from build123d import *

# Parameters (mm, degrees)
F0_R     = 25.4
F2_R     = 15.875
F4_R     = 15.875
F5_DEPTH = 50.8
F6_R     = 5.08
F7_DEPTH = 25.4
F8_DEPTH = 50.8
F9_R     = 5.08


with BuildPart() as f3:
    # F0 (on Top) → F3 section 0
    with BuildSketch(Plane.XY):
        Circle(F0_R)
    # F2 (on offset) → F3 section 1
    with BuildSketch(Plane.XY.offset(50.8)):
        Circle(F2_R)
    loft()

    # F4 (on face) → F5 (join)
    with BuildSketch(Plane.XY.offset(50.8)):
        Circle(F4_R)
    extrude(amount=F5_DEPTH)

    # F6 (on Front) → F7 (join)
    with BuildSketch(Plane.XZ):
        with Locations((0, 79.9094587564)):
            Circle(F6_R)
    extrude(amount=F7_DEPTH)

    # F8 (add): a face of the model
    f8_faces = [f3.faces().sort_by_distance(p)[0] for p in [
        (0, -25.4, 79.9094587564),
    ]]
    extrude(f8_faces, amount=-F8_DEPTH)

    # F9
    f9_edges = [f3.edges().sort_by_distance(p)[0] for p in [
        (-15.875, 0, 101.6),
    ]]
    fillet(f9_edges, radius=F9_R)

    # F10 (on Front) → F11 (revolve)
    with BuildSketch(Plane.XZ):
        Polygon((-15.8836290712, 107.9245372937), (0, 97.2370281816), (0, 139.7015303373), (-17.9440863431, 126.805588603), (-7.7806902118, 119.9670135975), align=None)
    revolve(axis=Axis((0, 0, 69.8507651687), (0, 0, 1)))


solid = f3.part
Geometry check sheet. Reference: the model listing, model coordinates, mm. A direction names the side the tool comes from. Coordinates: 2 decimals unless noted, no trailing zeros. Loops run counter-clockwise (first coordinate to the right, second up) from the corner with the lowest first, then second, coordinate; pieces in that order, holes last. Notation, with made-up numbers: (-1, 46.5) - (53, 46.5) arc R15 ccw to (53, 52.5) - close; hole circle Ø7 at (17.5, -23). An arc over 180 degrees is marked (long way). Use one line per item in the form item = value. Start each with the question number.
Item 1: Section check D-D, the plane z = 81.5. Enter the section's corners in (x, y) (3 decimals).
Item 2: Mould release check, pull along Z, two halves, no side actions. Record for faces 1 (the face through (-1.438, 2.765, 137.462)), 2 (the face through (0, 0, 0)), 3 (the face through (-5.075, 20.148, 80.133)): +Z half, -Z half, draft (parallel to the pull), parting line (faces both ways), or undercut.
Item 3: Section check B-B, the plane y = -9. Give the number of separate pieces and of enclosed holes in the cut face, and give its area (3 significant figures).
Item 4: Thickness scan on probe 1 along Z at (x, y) = (-15, 1.5); probe 2 along Z at (x, y) = (-9, 9.5); probe 3 along Y at (x, z) = (12.5, 31). Record the ranges inside material, lowest first.
Item 5: Gauge pin test, flat ends, axial feed: pin 1 (10 mm diameter, centred on x = -16.5, z = 63.5, fed in from -Y); pin 2 (4 mm diameter, centred on x = 18.5, y = 0.5, fed in from +Z); pin 3 (6.5 mm diameter, centred on x = 3, y = -2, fed in from +Z). Record the tip position at first contact, or that the pin passes through.
Item 6: Tool access check on faces 4 (the face through (-5.075, -20.148, 80.133)), 5 (the face through (6.57, 5.03, 120.3)), 6 (the face through (0, -25.4, 80)). Record the directions out of +Z, -Z, +X, -X, +Y, -Y that give a thin tool (end or side, any length) a straight path to the whole face; none if there is none.
Item 7: Section check A-A, the plane z = 24. Enter the section's corners in (x, y).
Computed:
q1.outline = (-4.825, -25.4) - (4.825, -25.4) - (4.825, -15.124) arc R15.875 ccw to (4.825, 15.124) - (4.825, 25.4) - (-4.825, 25.4) - (-4.825, 15.124) arc R15.875 ccw to (-4.825, -15.124) - close
q2.face_1 = +Z half
q2.face_2 = -Z half
q2.face_3 = undercut
q3.separate_pieces = 3
q3.enclosed_holes = 0
q3.area = 3,680 mm2
q4.probe_1 = 0 to 99.26, 107.38 to 109.13, 124.87 to 128.87
q4.probe_2 = 0 to 101.05, 106.04 to 112.08, 123.54 to 130.3
q4.probe_3 = -15.08 to 15.08
q5.pin_1 = -10.94
q5.pin_2 = 127.84
q5.pin_3 = 139.45
q6.face_4 = -Y
q6.face_5 = none
q6.face_6 = +Z, -Z, +X, -X, -Y
q7.outline = circle Ø41.8 at (0, 0)
